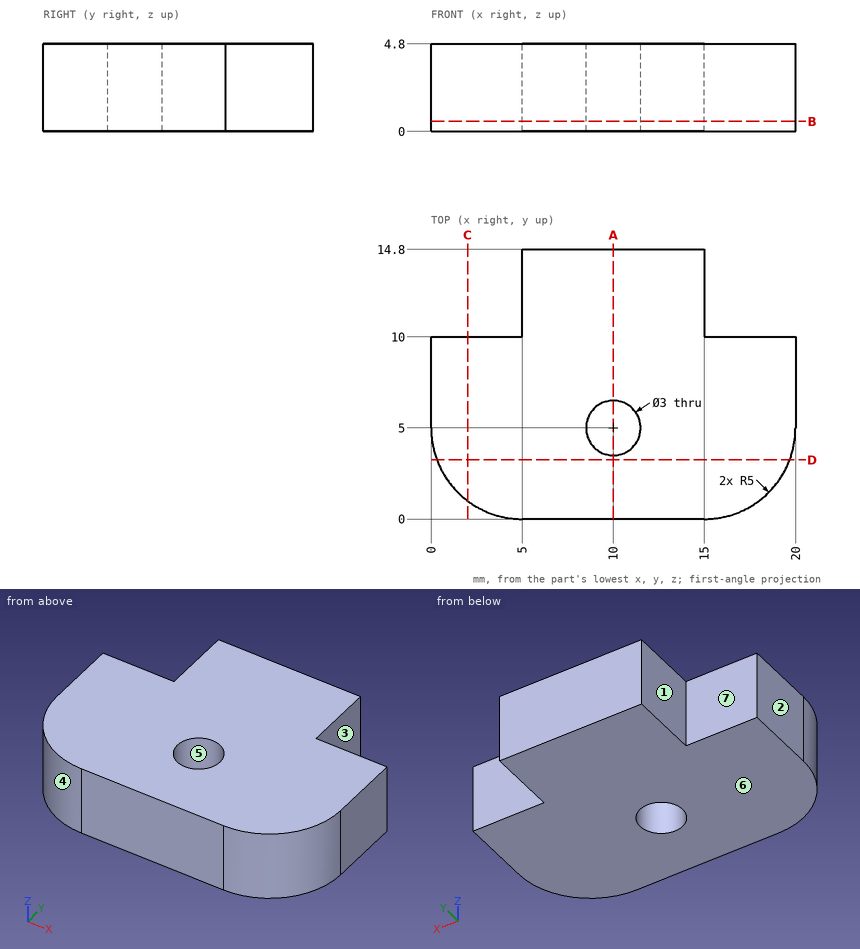
Here's the drawing with two shaded views (mm, measured from the low corner). I have some questions. A direction names the side the tool comes from. Coordinates: 2 decimals unless noted, no trailing zeros. Loops run counter-clockwise (first coordinate to the right, second up) from the corner with the lowest first, then second, coordinate; pieces in that order, holes last. Notation, with made-up numbers: (70.25, 82) -> (108.25, 82) arc R15 cw to (108.25, 91) -> close; hole circle Ø3 at (-16.5, 41). An arc over 180 degrees is marked (long way). Answer in a Markdown table with one row per item.
(1) If I drill on probe 1 along Y at (x, z) = (10, 3.05); probe 2 along X at (y, z) = (13, 4.25); probe 3 along X at (y, z) = (3.25, 1.3), over which ranges is the centre line in solid material (lowest first)?
Results found:
| item | result |
|---|---|
| probe 1 | y = 0 to 3.5, 6.5 to 14.8 |
| probe 2 | x = 5 to 15 |
| probe 3 | x = 0.32 to 19.68 |
(2) Imagine slicing it at C-C (x = 2). List the corners of the cut face in (y, z) for me.
Results found:
| item | result |
|---|---|
| outline | (1, 0) -> (10, 0) -> (10, 4.8) -> (1, 4.8) -> close |
(3) For the marked faces 1, 2 and 3, which set-ups out of +Z, -Z, +X, -X, +Y, -Y let a thin tool reach every point of the face, with its end or its side?
Results found:
| item | result |
|---|---|
| face 1 | +Z, -Z, -X, +Y |
| face 2 | +Z, -Z, -X, +Y, -Y |
| face 3 | +Z, -Z, +X, +Y |
(4) Imagine slicing it at D-D (y = 3.25). List the corners of the cut face in (x, z) for me.
Results found:
| item | result |
|---|---|
| outline | (0.32, 0) -> (19.68, 0) -> (19.68, 4.8) -> (0.32, 4.8) -> close |
(5) Imagine slicing it at A-A (x = 10). List the corners of the cut face in (y, z) for me, plus the area to 3 significant figures.
Results found:
| item | result |
|---|---|
| outline | (0, 0) -> (3.5, 0) -> (3.5, 4.8) -> (0, 4.8) -> close; (6.5, 0) -> (14.8, 0) -> (14.8, 4.8) -> (6.5, 4.8) -> close |
| area | 56.6 mm^2 |
(6) Imagine slicing it at B-B (z = 0.55). List the corners of the cut face in (x, y) for me, plus the area to 3 significant figures.
Results found:
| item | result |
|---|---|
| outline | (0, 5) arc R5 ccw to (5, 0) -> (15, 0) arc R5 ccw to (20, 5) -> (20, 10) -> (15, 10) -> (15, 14.8) -> (5, 14.8) -> (5, 10) -> (0, 10) -> close; hole circle Ø3 at (10, 5) |
| area | 230 mm^2 |
(7) Thinking about a two-plate mould opening in Y: for the marked faces 4, 5, 6 and 7, which applies, released by +Y, released by -Y, zero draft, split by the parting line, or undercut?
Results found:
| item | result |
|---|---|
| face 4 | released by -Y |
| face 5 | undercut |
| face 6 | zero draft |
| face 7 | released by +Y |
(8) Will these pins go through, and if not, where does the flat tip stop? pin 1 Ø1.5 at (x, z) = (16, 2) entering from -Y; pin 2 Ø5 at (x, y) = (17.5, 12) entering from -Z.
Results found:
| item | result |
|---|---|
| pin 1 | stops at y = 0.01 |
| pin 2 | stops at z = 0 |
